from build123d import *

# Parameters (mm, degrees)
BOSS_EXTRUDE1_DEPTH                         = 70.04
CSK_FOR_1_4_FLAT_HEAD_MACHINE_SCREW_2_COUNT = 2
CSK_FOR_1_4_FLAT_HEAD_MACHINE_SCREW_2_PITCH = 30
CUT_EXTRUDE2_REACH                          = 4.54
SKETCH8_R                                   = 6.6772536


with BuildPart() as part:
    # Sketch1 → Boss-Extrude1 (new body)
    with BuildSketch(Plane.XY.offset(12.7)):
        with BuildLine():
            Line((-3.81, 9.9314), (-3.81, -9.9314))
            ThreePointArc((-3.81, -9.9314), (-3.698407684, -10.200807684), (-3.429, -10.3124))
            Line((-3.429, -10.3124), (-0.381, -10.3124))
            ThreePointArc((-0.381, -10.3124), (-0.111592316, -10.200807684), (0, -9.9314))
            Line((0, -9.9314), (0, -3.556))
            ThreePointArc((0, -3.556), (0.111592316, -3.286592316), (0.381, -3.175))
            Line((0.381, -3.175), (2.159, -3.175))
            ThreePointArc((2.159, -3.175), (2.428407684, -3.063407684), (2.54, -2.794))
            Line((2.54, -2.794), (2.54, 2.794))
            ThreePointArc((2.54, 2.794), (2.428407684, 3.063407684), (2.159, 3.175))
            Line((2.159, 3.175), (0.381, 3.175))
            ThreePointArc((0.381, 3.175), (0.111592316, 3.286592316), (0, 3.556))
            Line((0, 3.556), (0, 9.9314))
            ThreePointArc((0, 9.9314), (-0.111592316, 10.200807684), (-0.381, 10.3124))
            Line((-0.381, 10.3124), (-3.429, 10.3124))
            ThreePointArc((-3.429, 10.3124), (-3.698407684, 10.200807684), (-3.81, 9.9314))
        make_face()
    extrude(amount=-BOSS_EXTRUDE1_DEPTH)

    # Sketch7 → CSK for 1/4 Flat Head Machine Screw (100)1 (revolve, cut)
    with BuildSketch(Plane(origin=(0, 0, -37.32), x_dir=(0, 0, -1), z_dir=(0, 1, 0))):
        Polygon((0, 0), (0, 3.81), (3.3782, 3.81), (3.3782, 2.768234659), (6.6772536, 0), align=None)
    csk_for_1_4_flat_head_machine_screw_100 = revolve(axis=Axis((6.35, 0, -37.32), (-1, 0, 0)), mode=Mode.SUBTRACT)

    # CSK for 1_4 Flat Head Machine Screw  2: CSK for 1/4 Flat Head Machine Screw (100)1 ×2
    with Locations(*[(0, 0, i * CSK_FOR_1_4_FLAT_HEAD_MACHINE_SCREW_2_PITCH) for i in range(1, CSK_FOR_1_4_FLAT_HEAD_MACHINE_SCREW_2_COUNT)]):
        add(csk_for_1_4_flat_head_machine_screw_100, mode=Mode.SUBTRACT)

    # Sketch8 → Cut-Extrude2 (cut, up to next)
    with BuildSketch(Plane(origin=(0, 0, 0), x_dir=(0, 0, -1), z_dir=(1, 0, 0)), mode=Mode.PRIVATE) as cut_extrude2_sk1:
        with Locations((7.32, 0)):
            Circle(SKETCH8_R)
    cut_extrude2_tool1 = extrude(cut_extrude2_sk1.sketch, amount=CUT_EXTRUDE2_REACH, mode=Mode.PRIVATE) & part.part
    add(cut_extrude2_tool1.solids().sort_by_distance((0, 0, -7.32))[0], mode=Mode.SUBTRACT)
    # Sketch8 → Cut-Extrude2 (cut, up to next)
    with BuildSketch(Plane(origin=(0, 0, 0), x_dir=(0, 0, -1), z_dir=(1, 0, 0)), mode=Mode.PRIVATE) as cut_extrude2_sk2:
        with Locations((37.32, 0)):
            Circle(SKETCH8_R)
    cut_extrude2_tool2 = extrude(cut_extrude2_sk2.sketch, amount=CUT_EXTRUDE2_REACH, mode=Mode.PRIVATE) & part.part
    add(cut_extrude2_tool2.solids().sort_by_distance((0, 0, -37.32))[0], mode=Mode.SUBTRACT)


solid = part.part
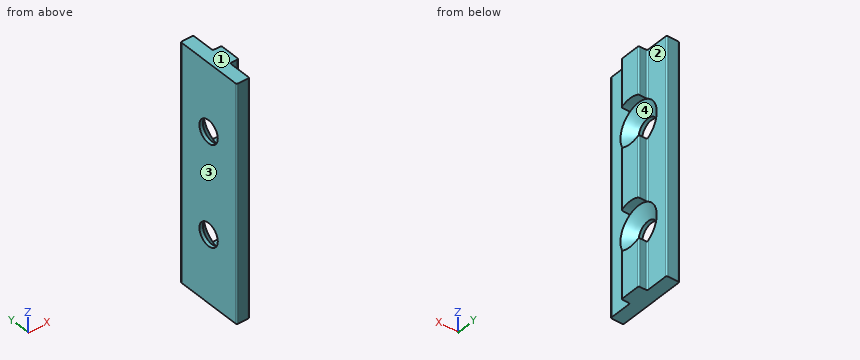
Part model, mm, in its own coordinate system. Face numbers are marked on the shaded views. A direction names the side the tool comes from. Coordinates: 2 decimals unless noted, no trailing zeros. Loops run counter-clockwise (first coordinate to the right, second up) from the corner with the lowest first, then second, coordinate; pieces in that order, holes last. Notation, with made-up numbers: M 80.5,68.5 L 90.5,68.5 A18 ccw 90.5,79.5 Z; hole C 47.25,41 d10. An arc over 180 degrees is marked long. Use a Markdown table: item, result. Add a question column.
Q1. Cut at C-C (x = 1.25). Write the cut outline in (y, z) (1 decimal).
Q2. Cut at D-D (z = -50.5). Write the cut outline in (x, y) (3 decimals), and give its area (3 significant figures).
Q3. Mould opens along Y. For the marked faces 3 and 4 say: +Y half, -Y half, draft (parallel to the pull), parting line (faces both ways), or undercut.
Q4. Probe L1, parallel to Z at x = -3.45, y = 0; L2, parallel to Z at x = -0.5, y = 2.25; L3, parallel to Y at x = -3.4, z = -37.32. List the from-to ranges inside material, lowest first.
Q5. Cut at A-A (y = 0). Write the cut outline in (x, z).
Q6. Pin check, flat tips, straight feed: P1, Ø1.4, axis at x = 1.5, z = -49, coming from the -Y side (3 decimals); P2, Ø1, axis at x = 1, y = -7.5, coming from the +Z side; P3, Ø3, axis at y = 6.5, z = -32.5, coming from the +X side; P4, Ø5, axis at y = -1.5, z = -37.5, coming from the +X side. Stop position of each tip, or through.
Q7. Which spindle directions (+Z, -Z, +X, -X, +Y, -Y) get a long thin tool onto all of the face, cutting with end or side? Do the marked faces 1 and 2. Say none if no direction does.
Q8. Cut at B-B (z = -7.32). Write the cut outline in (x, y), and give its area (3 significant figures).
Worked out:
| question | item | result |
|---|---|---|
| 1 | outline | M -3.2,-57.3 L 3.2,-57.3 L 3.2,-43.2 A6.7 cw -3.2,-43.2 Z; M -3.2,-31.4 A6.7 cw 3.2,-31.4 L 3.2,-13.2 A6.7 cw -3.2,-13.2 Z; M -3.2,-1.4 A6.7 cw 3.2,-1.4 L 3.2,12.7 L -3.2,12.7 Z |
| 2 | outline | M -3.81,-9.931 A0.381 ccw -3.429,-10.312 L -0.381,-10.312 A0.381 ccw 0,-9.931 L 0,-3.556 A0.381 cw 0.381,-3.175 L 2.159,-3.175 A0.381 ccw 2.54,-2.794 L 2.54,2.794 A0.381 ccw 2.159,3.175 L 0.381,3.175 A0.381 cw 0,3.556 L 0,9.931 A0.381 ccw -0.381,10.312 L -3.429,10.312 A0.381 ccw -3.81,9.931 Z |
| 2 | area | 94.6 mm2 |
| 3 | face 3 | draft |
| 3 | face 4 | undercut |
| 4 | L1 | z = -57.34 to -40.7, -33.94 to -10.7, -3.94 to 12.7 |
| 4 | L2 | z = -57.34 to -42.97, -31.67 to -12.97, -1.67 to 12.7 |
| 4 | L3 | y = -10.31 to -3.38, 3.38 to 10.31 |
| 5 | outline | M -3.81,-57.34 L 2.54,-57.34 L 2.54,-44 L 0,-44 L -2.77,-40.7 L -3.81,-40.7 Z; M -3.81,-33.94 L -2.77,-33.94 L 0,-30.64 L 2.54,-30.64 L 2.54,-14 L 0,-14 L -2.77,-10.7 L -3.81,-10.7 Z; M -3.81,-3.94 L -2.77,-3.94 L 0,-0.64 L 2.54,-0.64 L 2.54,12.7 L -3.81,12.7 Z |
| 6 | P1 | stops at y = -3.175 |
| 6 | P2 | passes through |
| 6 | P3 | stops at x = 0 |
| 6 | P4 | stops at x = -2.24 |
| 7 | face 1 | +Z, +X, -X, +Y, -Y |
| 7 | face 2 | +Z, -Z, +X, +Y |
| 8 | outline | M -3.81,-9.93 A0.38 ccw -3.43,-10.31 L -0.38,-10.31 A0.38 ccw 0,-9.93 L 0,-6.68 L -2.77,-3.38 L -3.81,-3.38 Z; M -3.81,3.38 L -2.77,3.38 L 0,6.68 L 0,9.93 A0.38 ccw -0.38,10.31 L -3.43,10.31 A0.38 ccw -3.81,9.93 Z |
| 8 | area | 43.6 mm2 |
